Build history of the part. All positions in model axes, mm. A direction names the side the tool comes from. Round coordinates to 2 decimals unless told otherwise and drop trailing zeros. Write each loop counter-clockwise with the first axis right and the second up, starting at its lowest first coordinate (ties: lowest second). Pieces come first, ordered by that corner, then holes. Notation, with made-up numbers: M 37,-2.5 L 94,-2.5 A13 ccw 94,4.5 Z; hole C 59,-14 d7. An arc over 180 degrees is marked long. Use a Markdown table: item, result.
from build123d import *

# Parameters (mm, degrees)
EXTRUDE_1_DEPTH     = 25
SKETCH_2_R          = 9.75
CUT_EXTRUDE_1_DEPTH = 5
FILLET_2_R          = 5


with BuildPart() as part:
    # 草圖1 → 填料-伸長1 (new body)
    with BuildSketch(Plane.XY):
        Polygon((12.962962963, -21.018518519), (47.037037037, -21.018518519), (47.037037037, 18.981481481), (37.777777778, 18.981481481), (37.777777778, -13.055555556), (12.962962963, -13.055555556), (12.962962963, 28.981481481), (2.962962963, 28.981481481), (2.962962963, -21.018518519), align=None)
    extrude(amount=EXTRUDE_1_DEPTH)

    # 草圖2 → 除料-伸長1 (cut)
    with BuildSketch(Plane.ZY.offset(-2.962962963)):
        with Locations(Location((12.5, 17.139708428, 0), (0, 0, 270))):
            Circle(SKETCH_2_R)
    extrude(amount=-CUT_EXTRUDE_1_DEPTH, mode=Mode.SUBTRACT)

    # 圓角2
    # the kernel refuses this fillet: 5 mm, written as the material it takes off along each edge
    with BuildSketch(Plane(origin=(47.037037037, -33.518518519, 25), x_dir=(0, 0, -1), z_dir=(0, 1, 0))) as fillet_2_piece_1:
        with BuildLine():
            CenterArc((FILLET_2_R, FILLET_2_R), FILLET_2_R, 180, 90)
            Line((0, FILLET_2_R), (0, 0))
            Line((0, 0), (FILLET_2_R, 0))
        make_face()
    extrude(amount=65, mode=Mode.SUBTRACT)
    with BuildSketch(Plane(origin=(47.037037037, -33.518518519, 0), x_dir=(0, 0, 1), z_dir=(0, 1, 0))) as fillet_2_piece_2:
        with BuildLine():
            CenterArc((FILLET_2_R, -FILLET_2_R), FILLET_2_R, 90, 90)
            Line((0, -FILLET_2_R), (0, 0))
            Line((0, 0), (FILLET_2_R, 0))
        make_face()
    extrude(amount=65, mode=Mode.SUBTRACT)
    with BuildSketch(Plane(origin=(37.777777778, 31.481481481, 0), x_dir=(1, 0, 0), z_dir=(0, -1, 0))) as fillet_2_piece_3:
        with BuildLine():
            CenterArc((FILLET_2_R, FILLET_2_R), FILLET_2_R, 180, 90)
            Line((0, FILLET_2_R), (0, 0))
            Line((0, 0), (FILLET_2_R, 0))
        make_face()
    extrude(amount=44.537037037, mode=Mode.SUBTRACT)
    with BuildSketch(Plane(origin=(12.962962963, -13.055555556, 25), x_dir=(-1, 0, 0), z_dir=(0, 1, 0))) as fillet_2_piece_4:
        with BuildLine():
            CenterArc((FILLET_2_R, -FILLET_2_R), FILLET_2_R, 90, 90)
            Line((0, -FILLET_2_R), (0, 0))
            Line((0, 0), (FILLET_2_R, 0))
        make_face()
    extrude(amount=54.537037037, mode=Mode.SUBTRACT)
    with BuildSketch(Plane(origin=(12.962962963, -13.055555556, 0), x_dir=(-1, 0, 0), z_dir=(0, 1, 0))) as fillet_2_piece_5:
        with BuildLine():
            CenterArc((FILLET_2_R, FILLET_2_R), FILLET_2_R, 180, 90)
            Line((0, FILLET_2_R), (0, 0))
            Line((0, 0), (FILLET_2_R, 0))
        make_face()
    extrude(amount=54.537037037, mode=Mode.SUBTRACT)
    with BuildSketch(Plane(origin=(37.777777778, -13.055555556, 25), x_dir=(0, -1, 0), z_dir=(-1, 0, 0))) as fillet_2_piece_6:
        with BuildLine():
            CenterArc((FILLET_2_R, -FILLET_2_R), FILLET_2_R, 90, 90)
            Line((0, -FILLET_2_R), (0, 0))
            Line((0, 0), (FILLET_2_R, 0))
        make_face()
    extrude(amount=24.814814815, mode=Mode.SUBTRACT)
    with BuildSketch(Plane(origin=(37.777777778, -13.055555556, 0), x_dir=(0, -1, 0), z_dir=(-1, 0, 0))) as fillet_2_piece_7:
        with BuildLine():
            CenterArc((FILLET_2_R, FILLET_2_R), FILLET_2_R, 180, 90)
            Line((0, FILLET_2_R), (0, 0))
            Line((0, 0), (FILLET_2_R, 0))
        make_face()
    extrude(amount=24.814814815, mode=Mode.SUBTRACT)
    with BuildSketch(Plane(origin=(37.777777778, 31.481481481, 0), x_dir=(1, 0, 0), z_dir=(0, -1, 0))) as fillet_2_piece_8a_section:
        with BuildLine():
            CenterArc((FILLET_2_R, FILLET_2_R), FILLET_2_R, 180, 90)
            Line((0, FILLET_2_R), (0, 0))
            Line((0, 0), (FILLET_2_R, 0))
        make_face()
    fillet_2_piece_8a = extrude(amount=57.037037037, mode=Mode.PRIVATE)
    fillet_2_piece_8a = split(fillet_2_piece_8a, bisect_by=Plane(origin=(38.909753349, -13.055555556, 1.131975571), z_dir=(0, -1, 0)), keep=Keep.TOP, mode=Mode.PRIVATE)
    with BuildSketch(Plane(origin=(50.277777778, -13.055555556, 0), x_dir=(0, -1, 0), z_dir=(-1, 0, 0))) as fillet_2_piece_8b_section:
        with BuildLine():
            CenterArc((FILLET_2_R, FILLET_2_R), FILLET_2_R, 180, 90)
            Line((0, FILLET_2_R), (0, 0))
            Line((0, 0), (FILLET_2_R, 0))
        make_face()
    fillet_2_piece_8b = extrude(amount=37.314814815, mode=Mode.PRIVATE)
    fillet_2_piece_8b = split(fillet_2_piece_8b, bisect_by=Plane(origin=(37.777777778, -14.187531127, 1.131975571), z_dir=(1, 0, 0)), keep=Keep.TOP, mode=Mode.PRIVATE)
    fillet_2_piece_8 = fillet_2_piece_8a & fillet_2_piece_8b
    add(fillet_2_piece_8, mode=Mode.SUBTRACT)
    with BuildSketch(Plane(origin=(37.777777778, -13.055555556, 25), x_dir=(0, -1, 0), z_dir=(-1, 0, 0))) as fillet_2_piece_9a_section:
        with BuildLine():
            CenterArc((FILLET_2_R, -FILLET_2_R), FILLET_2_R, 90, 90)
            Line((0, -FILLET_2_R), (0, 0))
            Line((0, 0), (FILLET_2_R, 0))
        make_face()
    fillet_2_piece_9a = extrude(amount=37.314814815, mode=Mode.PRIVATE)
    fillet_2_piece_9a = split(fillet_2_piece_9a, bisect_by=Plane(origin=(12.962962963, -14.187531127, 23.868024429), z_dir=(-1, 0, 0)), keep=Keep.TOP, mode=Mode.PRIVATE)
    with BuildSketch(Plane(origin=(12.962962963, -25.555555556, 25), x_dir=(-1, 0, 0), z_dir=(0, 1, 0))) as fillet_2_piece_9b_section:
        with BuildLine():
            CenterArc((FILLET_2_R, -FILLET_2_R), FILLET_2_R, 90, 90)
            Line((0, -FILLET_2_R), (0, 0))
            Line((0, 0), (FILLET_2_R, 0))
        make_face()
    fillet_2_piece_9b = extrude(amount=67.037037037, mode=Mode.PRIVATE)
    fillet_2_piece_9b = split(fillet_2_piece_9b, bisect_by=Plane(origin=(11.830987392, -13.055555556, 23.868024429), z_dir=(0, -1, 0)), keep=Keep.TOP, mode=Mode.PRIVATE)
    fillet_2_piece_9 = fillet_2_piece_9a & fillet_2_piece_9b
    add(fillet_2_piece_9, mode=Mode.SUBTRACT)
    with BuildSketch(Plane(origin=(37.777777778, -13.055555556, 0), x_dir=(0, -1, 0), z_dir=(-1, 0, 0))) as fillet_2_piece_10a_section:
        with BuildLine():
            CenterArc((FILLET_2_R, FILLET_2_R), FILLET_2_R, 180, 90)
            Line((0, FILLET_2_R), (0, 0))
            Line((0, 0), (FILLET_2_R, 0))
        make_face()
    fillet_2_piece_10a = extrude(amount=37.314814815, mode=Mode.PRIVATE)
    fillet_2_piece_10a = split(fillet_2_piece_10a, bisect_by=Plane(origin=(12.962962963, -14.187531127, 1.131975571), z_dir=(-1, 0, 0)), keep=Keep.TOP, mode=Mode.PRIVATE)
    with BuildSketch(Plane(origin=(12.962962963, -25.555555556, 0), x_dir=(-1, 0, 0), z_dir=(0, 1, 0))) as fillet_2_piece_10b_section:
        with BuildLine():
            CenterArc((FILLET_2_R, FILLET_2_R), FILLET_2_R, 180, 90)
            Line((0, FILLET_2_R), (0, 0))
            Line((0, 0), (FILLET_2_R, 0))
        make_face()
    fillet_2_piece_10b = extrude(amount=67.037037037, mode=Mode.PRIVATE)
    fillet_2_piece_10b = split(fillet_2_piece_10b, bisect_by=Plane(origin=(11.830987392, -13.055555556, 1.131975571), z_dir=(0, -1, 0)), keep=Keep.TOP, mode=Mode.PRIVATE)
    fillet_2_piece_10 = fillet_2_piece_10a & fillet_2_piece_10b
    add(fillet_2_piece_10, mode=Mode.SUBTRACT)


solid = part.part
Q1. Drop a flat-ended pin along its axis: P1, Ø7.5, axis at x = 44.5, z = 10.5, coming from the +Y side. Give the stop position or say it passes through.
Response values:
| item | result |
|---|---|
| P1 | stops at y = 18.98 |
Q2. Cut at D-D on x = 9.5. Give the cut face in (y, z), and give its area (3 significant figures).
Response values:
| item | result |
|---|---|
| outline | M -21.02,0 L -18.06,0 A5 ccw -16.52,0.24 L 28.98,0.24 L 28.98,24.76 L -16.52,24.76 A5 ccw -18.06,25 L -21.02,25 Z |
| area | 1,230 mm2 |
Q3. Two-plate mould, pull along Z, no slides. Class faces 1 (the flat face through (25, -21.019, 12)), 2 (the flat face through (6, -1, 25)), 3 (the flat face through (7.963, 17, 13)): +Z half, -Z half, draft (parallel to the pull), parting line (faces both ways), or undercut.
Response values:
| item | result |
|---|---|
| face 1 | draft |
| face 2 | +Z half |
| face 3 | undercut |
Q4. Drill centre lines: L1, parallel to X at y = 10.5, z = 18.75; L2, parallel to Y at x = 35.5, z = 8; L3, parallel to Y at x = 42, z = 6.75. Where is each one in solid material? Low to high.
Response values:
| item | result |
|---|---|
| L1 | x = 7.96 to 12.96, 37.78 to 47.04 |
| L2 | y = -21.02 to -13.06 |
| L3 | y = -21.02 to 18.98 |
Q5. Which spindle directions (+Z, -Z, +X, -X, +Y, -Y) get a long thin tool onto all of the face, cutting with end or side? Do faces 4 (the cylindrical face through (5.43, 12.64, 3.85)), 5 (the flat face through (12.963, 8, 12)), 6 (the cylindrical face through (11.537, 5.134, 1.504)), 7 (the flat face through (42, 18.981, 12)), 8 (the cylindrical face through (23.079, -14.559, 23.574)). Say none if no direction does.
Response values:
| item | result |
|---|---|
| face 4 | -X |
| face 5 | +Z, -Z, +Y |
| face 6 | -Z, +Y |
| face 7 | +Z, -Z, +X, +Y |
| face 8 | +Z, +Y |
Q6. Cut at B-B on z = 12.5. Give the cut face in (x, y), and give its area (3 significant figures).
Response values:
| item | result |
|---|---|
| outline | M 2.96,-21.02 L 47.04,-21.02 L 47.04,18.98 L 37.78,18.98 L 37.78,-13.06 L 12.96,-13.06 L 12.96,28.98 L 2.96,28.98 L 2.96,26.89 L 7.96,26.89 L 7.96,7.39 L 2.96,7.39 Z |
| area | 970 mm2 |
Q7. Cut at C-C on x = 29. Give the cut face in (y, z), and give its area (3 significant figures).
Response values:
| item | result |
|---|---|
| outline | M -21.02,0 L -18.06,0 A5 ccw -13.06,5 L -13.06,20 A5 ccw -18.06,25 L -21.02,25 Z |
| area | 188 mm2 |
Q8. Cut at A-A on y = -8.5. Give the cut face in (x, z).
Response values:
| item | result |
|---|---|
| outline | M 2.96,0 L 7.96,0 A5 ccw 12.96,5 L 12.96,20 A5 ccw 7.96,25 L 2.96,25 Z; M 37.78,5 A5 ccw 42.41,0.01 A5 ccw 47.04,5 L 47.04,20 A5 ccw 42.04,25 L 37.78,25 Z |
